Check sheet for the modelled part. Datum: model origin and axes. Units: mm. A direction names the side the tool comes from. Give positions to 0.01 mm unless a question says otherwise; leave off trailing zeros. Write each loop counter-clockwise with the first axis right and the second up, starting at its lowest first coordinate (ties: lowest second). Pieces come first, ordered by that corner, then holes. Notation, with made-up numbers: M 36.25,57.25 L 95.25,57.25 A3 ccw 95.25,62.25 Z; hole C 38.5,-40 d2. An arc over 180 degrees is marked long. Write item = value, one per line. Start each with the question number.
1) Cross-section at C-C, the plane y = 18.5. Record the cut outline in (x, z), plus the area to 3 significant figures.
2) Cross-section at A-A, the plane z = 3. Record the cut outline in (x, y), plus the area to 3 significant figures.
3) Cross-section at D-D, the plane x = 12.25. Record the cut outline in (y, z), plus the area to 3 significant figures.
4) Mould release check, pull along X, two halves, no side actions. Record for faces 1 (the cylindrical face through (20.763, 7.721, 3.195)), 2 (the flat face through (-23.2, 0.75, 1.6)), 3 (the cylindrical face through (-14.85, 21.92, 3.04)): released by +X, released by -X, zero draft, split by the parting line, or undercut.
5) Go/stop test with flat-tipped pins: pin 1 (0.8 mm diameter, centred on y = 15, z = 1.5, fed in from +X); pin 2 (4 mm diameter, centred on x = -0.5, y = 12, fed in from +Z); pin 3 (1.8 mm diameter, centred on x = 20.5, z = 4.5, fed in from +Y). Record where each tip stops, or that it passes through.
6) Access from +Z, -Z, +X, -X, +Y, -Y to the whole of each face (thin tool, end or side, straight path). Record for faces 4 (the flat face through (-18.25, 4, 3)), 5 (the flat face through (-18.25, 15, 3)), 6 (the flat face through (18.25, 15, 3)), 7 (the cylindrical face through (12.2, 17, 3)).
7) Cross-section at B-B, the plane x = 22.25. Record the cut outline in (y, z).
8) Scan lines: line 1 along X through (y, z) = (7.5, 3); line 2 along X through (y, z) = (19, 5.2); line 3 along X through (y, z) = (8.25, 5.6). Record each from-to range of solid material in increasing order. Write a range as [from, to].
Autodesk Inventor part; units mm, degrees
ref_plane "YZ Plane" through (0, 0, 0) normal (1, 0, 0) x (0, 1, 0)
ref_plane "XZ Plane" through (0, 0, 0) normal (0, 1, 0) x (-1, 0, 0)
ref_plane "XY Plane" through (0, 0, 0) normal (0, 0, 1) x (1, 0, 0)
sketch "Sketch1" plane through (0, 0, 0) normal (0, 0, 1) x (1, 0, 0)
  line L0 (-18.25, 6.5) -> (18.25, 6.5)
  line L1 (18.25, 6.5) -> (18.25, -6.5)
  line L2 (18.25, -6.5) -> (-18.25, -6.5)
  line L3 (-18.25, -6.5) -> (-18.25, 6.5)
  line L4 (26.25, 14.5) -> (-26.25, 14.5)
  line L5 (-26.25, 14.5) -> (-26.25, -14.5)
  line L6 (-26.25, -14.5) -> (26.25, -14.5)
  line L7 (26.25, -14.5) -> (26.25, 14.5)
  line L8 (-26.25, 0.75) -> (-18.25, 0.75)
  line L9 (18.25, 0.75) -> (26.25, 0.75)
  point P0 (0, 0)
  dimension "d0" = 36.5
  dimension "d1" = 13
  dimension "d2" = 8
  dimension "d3" = 18.25
  dimension "d4" = 6.5
  dimension "d5" = 0.75
  dimension "d6" = 0.75
extrude "Extrusion1" add sketch "Sketch1" along normal blind 6 contours L3 L8 L5 L4 L7 L9 L1 L0
sketch "Sketch2" plane through (18.25, 0.75, 0) normal (0, -1, 0) x (1, 0, 0)
  line L0 (-44.5, 0) -> (-36.5, 0)
  line L1 (-36.5, 0) -> (-36.5, 6)
  line L2 (-44.5, 6) -> (-36.5, 6)
  line L3 (-44.5, 0) -> (-44.5, 6)
  line L4 (0, 0) -> (8, 0)
  line L5 (8, 0) -> (8, 6)
  line L6 (0, 6) -> (8, 6)
  line L7 (0, 0) -> (0, 6)
  point P0 (-18.25, 0)
  point P1 (-40.5, 3)
  point P2 (4, 3)
  dimension "d9" = 8
  dimension "d10" = 6
  dimension "d11" = 3
  dimension "d12" = 4
  dimension "d13" = 4
  dimension "d14" = 3
hole "Hole1" at (-22.25, 0.75, 3) at (22.25, 0.75, 3) direction (0, 1, 0) diameter 3 end through all
sketch "Sketch3" plane through (0, 0, 0) normal (0, 0, -1) x (-1, 0, 0)
  line L0 (18.25, 6.5) -> (-18.25, 6.5)
  line L1 (18.25, 0.75) -> (18.25, 6.5)
  line L2 (26.25, 0.75) -> (18.25, 0.75)
  line L3 (26.25, 14.5) -> (26.25, 0.75)
  line L4 (-26.25, 14.5) -> (26.25, 14.5)
  line L5 (-26.25, 0.75) -> (-26.25, 14.5)
  line L6 (-18.25, 0.75) -> (-26.25, 0.75)
  line L7 (-18.25, 6.5) -> (-18.25, 0.75)
  line L8 (-26.25, 14.5) -> (26.25, 14.5)
  line L9 (18.25, 14.5) -> (-18.25, 14.5)
  line L10 (-18.25, 14.5) -> (-18.25, 22.5)
  line L11 (-18.25, 22.5) -> (18.25, 22.5)
  line L12 (18.25, 22.5) -> (18.25, 14.5)
  point P0 (0, 0)
  point P1 (12.25, 18.5)
  point P2 (-12.25, 18.5)
  dimension "d22" = 36.5
  dimension "d23" = 8
  dimension "d24" = 8
  dimension "d25" = 6
  dimension "d26" = 6
  dimension "d27" = 4
  dimension "d28" = 4
extrude "Extrusion2" add sketch "Sketch3" against normal blind 6 contours L4 L10 L11 L12
hole "Hole2" at (-12.25, 18.5, 0) at (12.25, 18.5, 0) direction (0, 0, 1) diameter 3 end through all
chamfer "Chamfer1" distance 3 distance2 6 1 edges at (-18.25, 22.5, 3) measured on face at (-6.0833, 22.5, 2)
chamfer "Chamfer2" distance 3 distance2 6 1 edges at (18.25, 22.5, 3) measured on face at (-4.0833, 22.5, 2)
fillet "Fillet1" radius 4 4 edges at (18.25, 16.5, 3) (15.25, 22.5, 3) (-15.25, 22.5, 3) (-18.25, 16.5, 3)
sketch "Sketch4" plane through (0, 0, 6) normal (0, 0, 1) x (1, 0, 0)
  circle A0 centre (12.25, 18.5) radius 1.5
  circle A1 centre (-12.25, 18.5) radius 1.5
  arc A2 (-17.8277, 17.3446) -> (-18.25, 15.5557) centre (-14.25, 15.5557) ccw
  line L0 (-18.25, 15.5557) -> (-18.25, 14.5)
  line L1 (-18.25, 14.5) -> (-26.25, 14.5)
  line L2 (-26.25, 14.5) -> (-26.25, 0.75)
  line L3 (-26.25, 0.75) -> (-18.25, 0.75)
  line L4 (-18.25, 0.75) -> (-18.25, 6.5)
  line L5 (-18.25, 6.5) -> (18.25, 6.5)
  line L6 (18.25, 6.5) -> (18.25, 0.75)
  line L7 (18.25, 0.75) -> (26.25, 0.75)
  line L8 (26.25, 0.75) -> (26.25, 14.5)
  line L9 (26.25, 14.5) -> (18.25, 14.5)
  line L10 (18.25, 14.5) -> (18.25, 15.5557)
  arc A3 (18.25, 15.5557) -> (17.8277, 17.3446) centre (14.25, 15.5557) ccw
  line L11 (16.3556, 20.2889) -> (17.8277, 17.3446)
  arc A4 (16.3556, 20.2889) -> (12.7779, 22.5) centre (12.7779, 18.5) ccw
  line L12 (12.7779, 22.5) -> (-12.7779, 22.5)
  arc A5 (-12.7779, 22.5) -> (-16.3556, 20.2889) centre (-12.7779, 18.5) ccw
  line L13 (-17.8277, 17.3446) -> (-16.3556, 20.2889)
  line L14 (-18.25, 6.5) -> (18.25, 6.5)
  line L15 (-4, 6.5) -> (4, 6.5)
  line L16 (4, 6.5) -> (4, 22.5)
  line L17 (4, 22.5) -> (-4, 22.5)
  line L18 (-4, 22.5) -> (-4, 6.5)
  point P0 (0, 0)
  dimension "d45" = 8
  dimension "d46" = 16
  dimension "d47" = 36.5
  dimension "d48" = 14.25
  dimension "d51" = 16
extrude "Extrusion3" cut sketch "Sketch4" against normal blind 1 contours L12 L16 L5 L18
equation "\"d46\" = d51"
equation "\"d48\" = -0.5 * d45 + 0.5 * d47"
properties part number "3DP_ABS_Electromagnet_Clamps" material "ABS Plastic"
Reply:
q1.outline = M -17.25,0 L -13.75,0 L -13.75,6 L -17.25,6 Z; M -10.75,0 L 10.75,0 L 10.75,6 L 4,6 L 4,5 L -4,5 L -4,6 L -10.75,6 Z; M 13.75,0 L 17.25,0 L 17.25,6 L 13.75,6 Z
q1.area = 163 mm2
q2.outline = M -26.25,0.75 L -23.75,0.75 L -23.75,14.5 L -26.25,14.5 Z; M -20.75,0.75 L -18.25,0.75 L -18.25,6.5 L 18.25,6.5 L 18.25,0.75 L 20.75,0.75 L 20.75,14.5 L 18.25,14.5 L 18.25,15.56 A4 ccw 17.83,17.34 L 16.36,20.29 A4 ccw 12.78,22.5 L -12.78,22.5 A4 ccw -16.36,20.29 L -17.83,17.34 A4 ccw -18.25,15.56 L -18.25,14.5 L -20.75,14.5 Z; M 23.75,0.75 L 26.25,0.75 L 26.25,14.5 L 23.75,14.5 Z; hole C -12.25,18.5 d3; hole C 12.25,18.5 d3
q2.area = 687 mm2
q3.outline = M 6.5,0 L 17,0 L 17,6 L 6.5,6 Z; M 20,0 L 22.5,0 L 22.5,6 L 20,6 Z
q3.area = 78.0 mm2
q4.face_1 = undercut
q4.face_2 = zero draft
q4.face_3 = released by -X
q5.pin_1 = 18.25
q5.pin_2 = 5
q5.pin_3 = 14.5
q6.face_4 = +Z, -Z, -Y
q6.face_5 = +Z, -Z, -X, +Y
q6.face_6 = +Z, -Z, +X, +Y
q6.face_7 = +Z, -Z
q7.outline = M 0.75,0 L 14.5,0 L 14.5,1.5 L 0.75,1.5 Z; M 0.75,4.5 L 14.5,4.5 L 14.5,6 L 0.75,6 Z
q8.line_1 = [-26.25, -23.75], [-20.75, 20.75], [23.75, 26.25]
q8.line_2 = [-17, -13.66], [-10.84, -4], [4, 10.84], [13.66, 17]
q8.line_3 = [-26.25, -4], [4, 26.25]
